Work out the finished part from the listing and answer in its coordinate system (mm). A direction names the side the tool comes from. Give positions to 0.01 mm unless a question says otherwise; leave off trailing zeros. Write each loop counter-clockwise with the first axis right and the second up, starting at its lowest first coordinate (ties: lowest second). Pieces come first, ordered by that corner, then holes.
1) Find section A-A (y = -1.5). Determine the outline of the cut face in (x, z).
2) Find section D-D (x = -31). Determine the outline of the cut face in (y, z), plus the area to 3 significant figures.
3) Find section C-C (z = 31.5). Determine the outline of the cut face in (x, y), plus the area to 3 significant figures.
4) Given pin 1 Ø19.5 at (x, z) = (-9.5, 34.5) entering from +Y; pin 2 Ø24 at (y, z) = (-0.5, 14) entering from -X; pin 3 Ø3 at (y, z) = (8, 13) entering from +X, each flat-ended and moving along its own axis, determine where each tip first touches the part or whether it passes through.
5) Find section B-B (x = -4). Determine the outline of the cut face in (y, z).
6) Straight lines are drawn through the part: probe 1 along Y at (x, z) = (-5.5, 44); probe 2 along Z at (x, y) = (-26, 25.5); probe 3 along X at (y, z) = (-4, 17). For each, find the intervals that lie inside material, in ascending order.
7) A tool of negligible diameter and unlimited length cuts with its end or side. For faces 1 (the face through (0, -15, 23)), 2 (the face through (-19.5, 0, 23)), 3 (the face through (19.5, 0, 23)), from which of +Z, -Z, +X, -X, +Y, -Y can it reach the whole face along a straight path? Write none if from no direction.
Autodesk Inventor part; units mm, degrees
ref_plane "YZ Plane" through (0, 0, 0) normal (1, 0, 0) x (0, 1, 0)
ref_plane "XZ Plane" through (0, 0, 0) normal (0, 1, 0) x (-1, 0, 0)
ref_plane "XY Plane" through (0, 0, 0) normal (0, 0, 1) x (1, 0, 0)
sketch "Skizze1" plane through (0, 0, 0) normal (0, 0, 1) x (1, 0, 0)
  line L0 (-19.5, -15) -> (19.5, -15)
  line L1 (19.5, -15) -> (19.5, 15)
  line L2 (19.5, 15) -> (-19.5, 15)
  line L3 (-19.5, 15) -> (-19.5, -15)
  line L4 (-19.5, -15) -> (19.5, 15) construction
  line L5 (19.5, -15) -> (-19.5, 15) construction
  point P0 (0, 0)
  point P1 (0, 0)
  point P2 (0, 0)
  dimension "d8" = 39
  dimension "d9" = 30
extrude "Extrusion1" add sketch "Skizze1" along normal blind 47
sketch "Skizze2" plane through (0, 0, 47) normal (0, 0, 1) x (1, 0, 0)
  line L0 (-40, -40) -> (40, -40)
  line L1 (40, -40) -> (40, 40)
  line L2 (40, 40) -> (-40, 40)
  line L3 (-40, 40) -> (-40, -40)
  point P0 (0, 0)
  point P1 (0, 40)
  point P2 (-40, 0)
  dimension "d4" = 80
extrude "Extrusion2" add sketch "Skizze2" along normal blind 4
properties part number "Beacon-Support"
Results:
1. outline: (-40, 47) - (-19.5, 47) - (-19.5, 0) - (19.5, 0) - (19.5, 47) - (40, 47) - (40, 51) - (-40, 51) - close
2. outline: (-40, 47) - (40, 47) - (40, 51) - (-40, 51) - close
2. area: 320 mm2
3. outline: (-19.5, -15) - (19.5, -15) - (19.5, 15) - (-19.5, 15) - close
3. area: 1,170 mm2
4. pin 1: stops at y = 15
4. pin 2: stops at x = -19.5
4. pin 3: stops at x = 19.5
5. outline: (-40, 47) - (-15, 47) - (-15, 0) - (15, 0) - (15, 47) - (40, 47) - (40, 51) - (-40, 51) - close
6. probe 1: y = -15 to 15
6. probe 2: z = 47 to 51
6. probe 3: x = -19.5 to 19.5
7. face 1: -Z, +X, -X, -Y
7. face 2: -Z, -X, +Y, -Y
7. face 3: -Z, +X, +Y, -Y
